```python
from build123d import *

# Parameters (mm, degrees)
F0_R      = 5.15
F1_DEPTH  = 9.3
F2_W      = 1.2
F2_H      = 13.8570601121
F3_DEPTH  = 9.301
F4_W      = 3.5
F4_H      = 0.9
F5_DEPTH  = 25
F7_R      = 1.6
F8_DEPTH  = 21.151
F10_DEPTH = 25
F12_DEPTH = 25
F13_R     = 0.5


with BuildPart() as f1:
    # F0 (on Top) → F1 (new body)
    with BuildSketch(Plane.XY):
        with BuildLine():
            ThreePointArc((3, -7.5777635223), (6.7406416609, -4.5810752013), (8.15, 0))
            ThreePointArc((8.15, 0), (-4.5810752013, 6.7406416609), (-3, -7.5777635223))
            Line((-3, -7.5777635223), (3, -7.5777635223))
        make_face()
        Circle(F0_R, mode=Mode.SUBTRACT)
        with BuildLine():
            Line((3, -7.5777635223), (-3, -7.5777635223))
            ThreePointArc((-3, -7.5777635223), (0, -8.15), (3, -7.5777635223))
        make_face()
        with BuildLine():
            ThreePointArc((3, -7.5777635223), (0, -8.15), (-3, -7.5777635223))
            Line((-3, -7.5777635223), (-3, -11.0777635223))
            Line((-3, -11.0777635223), (3, -11.0777635223))
            Line((3, -11.0777635223), (3, -7.5777635223))
        make_face()
    extrude(amount=F1_DEPTH)

    # F2 (on Top) → F3 (cut, through all)
    with BuildSketch(Plane.XY):
        with Locations((0, -6.928530056)):
            Rectangle(F2_W, F2_H)
    extrude(amount=F3_DEPTH, mode=Mode.SUBTRACT)

    # F4 (on face) → F5 (cut)
    with BuildSketch(Plane(origin=(-3, 0, 0), x_dir=(0, -1, 0), z_dir=(-1, 0, 0))):
        with Locations((9.3277635223, 8.85)):
            Rectangle(F4_W, F4_H)
        with Locations((9.3277635223, 0.45)):
            Rectangle(F4_W, F4_H)
    extrude(amount=-F5_DEPTH, mode=Mode.SUBTRACT)

    # F7 (on offset) → F8 (cut, through all)
    with BuildSketch(Plane(origin=(-13, 0, 0), x_dir=(0, -1, 0), z_dir=(-1, 0, 0))):
        with Locations((8.0777635223, 4.65)):
            Circle(F7_R)
    extrude(amount=-F8_DEPTH, mode=Mode.SUBTRACT)

    # F9 (on face) → F10 (cut)
    with BuildSketch(Plane(origin=(-3, 0, 0), x_dir=(0, -1, 0), z_dir=(-1, 0, 0))):
        Polygon((10.8127635223, 6.2290529862), (8.0777635223, 7.8081059725), (5.3427635223, 6.2290529862), (5.3427635223, 3.0709470138), (8.0777635223, 1.4918940275), (10.8127635223, 3.0709470138), align=None)
    extrude(amount=F10_DEPTH, mode=Mode.SUBTRACT)

    # F11 (on face) → F12 (cut)
    with BuildSketch(Plane.YZ.offset(3)):
        Polygon((-5.3427635223, 3.0709470138), (-5.3427635223, 6.2290529862), (-8.0777635223, 7.8081059725), (-10.8127635223, 6.2290529862), (-10.8127635223, 3.0709470138), (-8.0777635223, 1.4918940275), align=None)
    extrude(amount=F12_DEPTH, mode=Mode.SUBTRACT)

    # F13
    f13_edges = [f1.edges().sort_by_distance(p)[0] for p in [
        (0, 8.15, 9.3),
        (3, -9.327764, 8.4),
        (-3, -9.327764, 8.4),
        (-1.8, -7.577764, 9.3),
        (1.8, -7.577764, 9.3),
        (1.8, -11.077764, 8.4),
        (-1.8, -11.077764, 8.4),
    ]]
    fillet(f13_edges, radius=F13_R)


solid = f1.part
```
Build history of the part. All positions in model axes, mm. A direction names the side the tool comes from. Give positions to 0.01 mm unless a question says otherwise; leave off trailing zeros. Loops run counter-clockwise (first coordinate to the right, second up) from the corner with the lowest first, then second, coordinate; pieces in that order, holes last. Notation, with made-up numbers: (27, -17) -> (47, -17) arc R33 ccw to (47, 22) -> close; hole circle Ø10 at (65, 75). An arc over 180 degrees is marked (long way). One line per question, with ' | ' between items.
Q1. Pull direction Z, two halves, no side cores. Call faces 1 (the flat face through (1.8, -7.578, 0.4)), 2 (the flat face through (2, -9, 0.9)), 3 (the flat face through (3, -10, 4)), 4 (the flat face through (-2, -9, 8.4)): pulls with the +Z half, pulls with the -Z half, needs draft (parallel to the pull), parting line crosses it, or undercut.
Filled sheet:
face 1: needs draft | face 2: pulls with the -Z half | face 3: undercut | face 4: pulls with the +Z half
Q2. Cut at C-C, the plane z = 7.25. Write the cut outline in (x, y).
Filled sheet:
outline: (-3.98, -7.11) -> (-3, -7.11) -> (-3, -11.08) -> (-0.6, -11.08) -> (-0.6, -5.11) arc R5.15 cw (long way) to (0.6, -5.11) -> (0.6, -11.08) -> (3, -11.08) -> (3, -7.11) -> (3.98, -7.11) arc R8.15 ccw (long way) to start
Q3. Drill centre lines: line 1 along Y through (x, z) = (-1.95, 4.65); line 2 along X through (y, z) = (0, 7.75); line 3 along Y through (x, z) = (2, 3.5). Where is each one in solid material? Low to high. Write a range as [from, to].
Filled sheet:
line 1: y = [-11.08, -9.68], [-6.48, -4.77], [4.77, 7.91] | line 2: x = [-8.15, -5.15], [5.15, 8.15] | line 3: y = [-11.08, -9.19], [-6.97, -4.75], [4.75, 7.9]
Q4. Cut at B-B, the plane x = -2. Count the separate pieces of the cut face and the enclosed holes in it, plus the area to 3 significant figures.
Filled sheet:
separate pieces: 2 | enclosed holes: 1 | area: 73.7 mm²
Q5. Drop flat-ended pins along their axis: pin 1 (1.7 mm diameter, centred on y = -9.5, z = 3, fed in from +X); pin 2 (0.7 mm diameter, centred on x = 2.5, z = 0, fed in from -Y); pin 3 (3 mm diameter, centred on x = -4.5, y = -4, fed in from -Z); pin 4 (1.7 mm diameter, centred on y = -8.5, z = 4.5, fed in from -X). Give the stop position or say it passes through.
Filled sheet:
pin 1: stops at x = 3 | pin 2: stops at y = -7.58 | pin 3: stops at z = 0 | pin 4: passes through
Q6. Cut at A-A, the plane z = 4.65. Write the cut outline in (x, y).
Filled sheet:
outline: (-6.15, -5.34) -> (-3, -5.34) -> (-3, -6.48) -> (-0.6, -6.48) -> (-0.6, -5.11) arc R5.15 cw (long way) to (0.6, -5.11) -> (0.6, -6.48) -> (3, -6.48) -> (3, -5.34) -> (6.15, -5.34) arc R8.15 ccw (long way) to start; (-3, -11.08) -> (-0.6, -11.08) -> (-0.6, -9.68) -> (-3, -9.68) -> close; (0.6, -11.08) -> (3, -11.08) -> (3, -9.68) -> (0.6, -9.68) -> close
Q7. Tool access for faces 5 (the flat face through (4.205, -6.196, 6.722)), 6 (the flat face through (-0.6, -6, 5)), 7 (the flat face through (-5, -5.343, 5)): list every direction of +Z, -Z, +X, -X, +Y, -Y with a clear straight run to the whole face (end or side of a thin tool).
Filled sheet:
face 5: +X, -Y | face 6: +Z, -Z, -Y | face 7: -X, -Y
